Geometry: final body of the model. Coordinates: model frame, mm. Face numbers are marked on the shaded views. A direction names the side the tool comes from. Give positions to 0.01 mm unless a question says otherwise; leave off trailing zeros. Write each loop counter-clockwise with the first axis right and the second up, starting at its lowest first coordinate (ties: lowest second). Pieces come first, ordered by that corner, then holes.
Q1. Pin query (flat end, axial travel): pin 1 (11.5 mm diameter, centred on y = 25.5, z = 5.5, fed in from -X); pin 2 (12 mm diameter, centred on y = 62, z = -4, fed in from -X); pin 3 (1.5 mm diameter, centred on x = 6, y = 41.5, fed in from +Z); pin 4 (9.5 mm diameter, centred on x = 0, z = 0, fed in from -Y). Return the tip coordinate at first contact, or that it passes through.
Q2. Cut plane C-C on x = 0. Return the cut outline in (y, z), plus the area to 3 significant figures.
Q3. Line query: L1, parallel to X at y = 39, z = 0; L2, parallel to X at y = 41, z = 0; L3, parallel to Y at x = -8.25, z = 7. Output: solid intervals per line, ascending.
Q4. Reachability of the marked faces 1, 2, 3 and 4 from +Z, -Z, +X, -X, +Y, -Y: full face, straight path, thin tool, end or side. Return the list, or none.
Q5. Draft query along Z for the marked faces 5, 6, 7 and 8. Return one class per face: pulls with the +Z half, pulls with the -Z half, needs draft (parallel to the pull), parting line crosses it, or undercut.
Q6. Cut plane A-A on z = 0. Return the cut outline in (x, y).
Q7. Cut plane D-D on y = 7. Return the cut outline in (x, z), plus the area to 3 significant figures.
Q8. Cut plane B-B on y = 32.5. Return the cut outline in (x, z), plus the area to 3 significant figures.
```python
from build123d import *

# Parameters (mm, degrees)
SKETCH1_W           = 30
SKETCH1_H           = 30
BOSS_EXTRUDE1_DEPTH = 40
SKETCH2_R           = 9
BOSS_EXTRUDE2_DEPTH = 30
SKETCH3_R           = 6
CUT_EXTRUDE1_DEPTH  = 60
SKETCH4_W           = 23
SKETCH4_H           = 37
CUT_EXTRUDE2_DEPTH  = 5
SKETCH5_W           = 23
SKETCH5_H           = 37
CUT_EXTRUDE3_DEPTH  = 5


with BuildPart() as part:
    # Sketch1 → Boss-Extrude1 (new body)
    with BuildSketch(Plane(origin=(0, 0, 0), x_dir=(1, 0, 0), z_dir=(0, 1, 0))):
        Rectangle(SKETCH1_W, SKETCH1_H)
    extrude(amount=BOSS_EXTRUDE1_DEPTH)

    # Sketch2 → Boss-Extrude2 (add)
    with BuildSketch(Plane(origin=(0, 40, 0), x_dir=(1, 0, 0), z_dir=(0, 1, 0))):
        with Locations(Location((0, 0, 0), (0, 0, 270))):
            Circle(SKETCH2_R)
    extrude(amount=BOSS_EXTRUDE2_DEPTH)

    # Sketch3 → Cut-Extrude1 (cut)
    with BuildSketch(Plane(origin=(0, 70, 0), x_dir=(1, 0, 0), z_dir=(0, 1, 0))):
        with Locations(Location((0, 0, 0), (0, 0, 270))):
            Circle(SKETCH3_R)
    extrude(amount=-CUT_EXTRUDE1_DEPTH, mode=Mode.SUBTRACT)

    # Sketch4 → Cut-Extrude2 (cut)
    with BuildSketch(Plane(origin=(15, 0, 0), x_dir=(0, 0, -1), z_dir=(1, 0, 0))):
        with Locations((0, 18.5)):
            Rectangle(SKETCH4_W, SKETCH4_H)
    extrude(amount=-CUT_EXTRUDE2_DEPTH, mode=Mode.SUBTRACT)

    # Sketch5 → Cut-Extrude3 (cut)
    with BuildSketch(Plane.ZY.offset(15)):
        with Locations((0, 18.5)):
            Rectangle(SKETCH5_W, SKETCH5_H)
    extrude(amount=-CUT_EXTRUDE3_DEPTH, mode=Mode.SUBTRACT)


solid = part.part
```
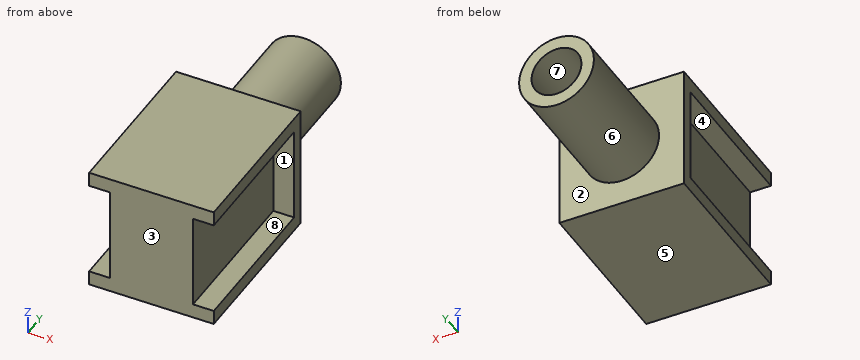
Data:
1. pin 1: stops at x = -10
1. pin 2: stops at x = -9
1. pin 3: stops at z = 7.31
1. pin 4: stops at y = 0
2. outline: (0, -15) - (40, -15) - (40, -9) - (70, -9) - (70, -6) - (10, -6) - (10, 6) - (70, 6) - (70, 9) - (40, 9) - (40, 15) - (0, 15) - close
2. area: 1,020 mm2
3. L1: x = -15 to -6, 6 to 15
3. L2: x = -9 to -6, 6 to 9
3. L3: y = 0 to 40
4. face 1: +X, -Y
4. face 2: +Y
4. face 3: +Z, -Z, +X, -X, -Y
4. face 4: -X, -Y
5. face 5: pulls with the -Z half
5. face 6: parting line crosses it
5. face 7: undercut
5. face 8: undercut
6. outline: (-15, 37) - (-10, 37) - (-10, 0) - (10, 0) - (10, 37) - (15, 37) - (15, 40) - (9, 40) - (9, 70) - (6, 70) - (6, 10) - (-6, 10) - (-6, 70) - (-9, 70) - (-9, 40) - (-15, 40) - close
7. outline: (-15, -15) - (15, -15) - (15, -11.5) - (10, -11.5) - (10, 11.5) - (15, 11.5) - (15, 15) - (-15, 15) - (-15, 11.5) - (-10, 11.5) - (-10, -11.5) - (-15, -11.5) - close
7. area: 670 mm2
8. outline: (-15, -15) - (15, -15) - (15, -11.5) - (10, -11.5) - (10, 11.5) - (15, 11.5) - (15, 15) - (-15, 15) - (-15, 11.5) - (-10, 11.5) - (-10, -11.5) - (-15, -11.5) - close; hole circle Ø12 at (0, 0)
8. area: 557 mm2
